Check sheet for the modelled part. Datum: model origin and axes. Units: mm. Coordinates: 2 decimals unless noted, no trailing zeros. Write each loop counter-clockwise with the first axis right and the second up, starting at its lowest first coordinate (ties: lowest second). Pieces come first, ordered by that corner, then holes. Notation, with made-up numbers: (-15, 82) -> (25, 82) arc R28 ccw to (25, 121) -> close; hole circle Ø10 at (5, 37.5). An arc over 180 degrees is marked (long way). Put each result on its own line as item: value.
```python
from build123d import *

# Parameters (mm, degrees)
SKETCH1_W           = 500
SKETCH1_H           = 500
BOSS_EXTRUDE1_DEPTH = 1000
CUT_EXTRUDE1_REACH  = 1147.644


with BuildPart() as part:
    # Sketch1 → Boss-Extrude1 (new body)
    with BuildSketch(Plane(origin=(0, 0, 0), x_dir=(1, 0, 0), z_dir=(0, 1, 0))):
        Rectangle(SKETCH1_W, SKETCH1_H)
    extrude(amount=BOSS_EXTRUDE1_DEPTH)

    # Sketch3 → Cut-Extrude1 (cut, up to next)
    with BuildSketch(Plane(origin=(250, 0, 0), x_dir=(0, 0, -1), z_dir=(1, 0, 0)), mode=Mode.PRIVATE) as cut_extrude1_sk1:
        Polygon((-250, 750), (0, 1000), (-250, 1000), align=None)
    cut_extrude1_tool1 = extrude(cut_extrude1_sk1.sketch, amount=-CUT_EXTRUDE1_REACH, mode=Mode.PRIVATE) & part.part
    add(cut_extrude1_tool1.solids().sort_by_distance((250, 916.666667, 166.666667))[0], mode=Mode.SUBTRACT)


solid = part.part
```
Q1. Cross-section at A-A (z = 122.5). Record the cut outline in (x, y).
Recorded:
outline: (-250, 0) -> (250, 0) -> (250, 877.5) -> (-250, 877.5) -> close
Q2. Cross-section at B-B (x = -174.5). Record the cut outline in (y, z).
Recorded:
outline: (0, -250) -> (1000, -250) -> (1000, 0) -> (750, 250) -> (0, 250) -> close
Q3. Material ranges on line 1 along Y through (x, z) = (-66.5, 37.5); line 2 along Z through (x, y) = (134.5, 815.5); line 3 along Y through (x, z) = (96, 157.5), recorded low to high.
Recorded:
line 1: y = 0 to 962.5
line 2: z = -250 to 184.5
line 3: y = 0 to 842.5
Q4. Depth check by flat-ended pin: P1, Ø1.5, axis at x = -123, z = 158.5, coming from the +Y side; P2, Ø6, axis at x = -171, y = 836, coming from the +Z side. Enter the tip coordinate at first touch or a pass-through.
Recorded:
P1: stops at y = 842.25
P2: stops at z = 167
Q5. Cross-section at C-C (y = 900). Record the cut outline in (x, z), plus the area to 3 significant figures.
Recorded:
outline: (-250, -250) -> (250, -250) -> (250, 100) -> (-250, 100) -> close
area: 175,000 mm2
